from build123d import *

# Parameters (mm, degrees)
SKETCH1_W               = 800
SKETCH1_H               = 800
SKETCH1_W_2             = 700
SKETCH1_H_2             = 700
BOSS_EXTRUDE1_DEPTH     = 50
SKETCH2_W               = 50
SKETCH2_H               = 50
BOSS_EXTRUDE2_DEPTH     = 800
CUT_EXTRUDE1_DEPTH      = 980.795897113
CUT_EXTRUDE1_DEPTH_BACK = 980.795897113
SKETCH3_R               = 5


with BuildPart() as part:
    # Sketch1 → Boss-Extrude1 (new body)
    with BuildSketch(Plane(origin=(0, 0, 0), x_dir=(1, 0, 0), z_dir=(0, 1, 0))):
        Rectangle(SKETCH1_W, SKETCH1_H)
        Rectangle(SKETCH1_W_2, SKETCH1_H_2, mode=Mode.SUBTRACT)
    extrude(amount=BOSS_EXTRUDE1_DEPTH)

    # Sketch2 → Boss-Extrude2 (add)
    with BuildSketch(Plane.XZ.offset(-50)):
        with Locations((-375, 375)):
            Rectangle(SKETCH2_W, SKETCH2_H)
        with Locations((375, 375)):
            Rectangle(SKETCH2_W, SKETCH2_H)
        with Locations((375, -375)):
            Rectangle(SKETCH2_W, SKETCH2_H)
        with Locations((-375, -375)):
            Rectangle(SKETCH2_W, SKETCH2_H)
    extrude(amount=BOSS_EXTRUDE2_DEPTH)

    # Sketch3 → Cut-Extrude1 (cut, two sides: drawn at the far end of the back side and taken through both)
    with BuildSketch(Plane(origin=(0, 50, 0), x_dir=(1, 0, 0), z_dir=(0, 1, 0)).offset(-CUT_EXTRUDE1_DEPTH_BACK)):
        with Locations(Location((-200, 375, 0), (0, 0, 90))):
            Circle(SKETCH3_R)
        with Locations(Location((-375, 200, 0), (0, 0, 90))):
            Circle(SKETCH3_R)
        with Locations(Location((-375, -200, 0), (0, 0, 90))):
            Circle(SKETCH3_R)
        with Locations(Location((-200, -375, 0), (0, 0, 90))):
            Circle(SKETCH3_R)
        with Locations(Location((200, -375, 0), (0, 0, 90))):
            Circle(SKETCH3_R)
        with Locations(Location((375, -200, 0), (0, 0, 90))):
            Circle(SKETCH3_R)
        with Locations(Location((375, 200, 0), (0, 0, 90))):
            Circle(SKETCH3_R)
        with Locations(Location((200, 375, 0), (0, 0, 90))):
            Circle(SKETCH3_R)
    extrude(amount=CUT_EXTRUDE1_DEPTH + CUT_EXTRUDE1_DEPTH_BACK, mode=Mode.SUBTRACT)


solid = part.part
CAD build for the part. Positions are in the model's coordinates, mm. A direction names the side the tool comes from. Round coordinates to 2 decimals unless told otherwise and drop trailing zeros. Order: outer loops, then holes, each group sorted by start corner. A loop starts at its lowest first (then second) coordinate and runs counter-clockwise, first axis right, second up. Notation, with made-up numbers: (67, 68) - (102, 68) arc R8 cw to (102, 77) - close; hole circle Ø7 at (-32.75, 3.25). An arc over 180 degrees is marked (long way). Return JSON: item names as keys, results as strings.
(1) Cut at A-A (y = -82). Give the cut face in (x, z).
Answer key:
{"outline": "(-400, -400) - (-350, -400) - (-350, -350) - (-400, -350) - close; (-400, 350) - (-350, 350) - (-350, 400) - (-400, 400) - close; (350, -400) - (400, -400) - (400, -350) - (350, -350) - close; (350, 350) - (400, 350) - (400, 400) - (350, 400) - close"}
(2) Pull direction Z, two halves, no side cores. Call faces 5 (the face through (-2, 4, -400)), 6 (the face through (-357, 50, -2)), 7 (the face through (-375, 0, -5)), 8 (the face through (350, 25, 5)): +Z half, -Z half, draft (parallel to the pull), parting line (faces both ways), or undercut.
Answer key:
{"face 5": "-Z half", "face 6": "draft", "face 7": "undercut", "face 8": "undercut"}
(3) Pin check, flat tips, straight feed: pin 1 Ø15 at (x, z) = (-371.5, -52.5) entering from -Y; pin 2 Ø11.5 at (x, z) = (-375, -200) entering from +Y. Stop position of each tip, or through.
Answer key:
{"pin 1": "stops at y = 0", "pin 2": "stops at y = 50"}
(4) Cut at B-B (z = 55). Give the cut face in (x, y), then the cut area to 3 significant figures.
Answer key:
{"outline": "(-400, 0) - (-350, 0) - (-350, 50) - (-400, 50) - close; (350, 0) - (400, 0) - (400, 50) - (350, 50) - close", "area": "5,000 mm^2"}
(5) Wall check: probe 1 along Z at (x, y) = (-375, 24); probe 2 along X at (y, z) = (-564, -351). Give the ranges that are in metal, low to high. Write a range as from..to.
Answer key:
{"probe 1": "z = -400..-205, -195..195, 205..400", "probe 2": "x = -400..-350, 350..400"}
(6) Tool access for faces 1 (the face through (350, -370, 375)), 2 (the face through (-5, 25, -350)), 3 (the face through (-2, 4, 400)), 4 (the face through (-375, -370, -350)): list every direction of +Z, -Z, +X, -X, +Y, -Y with a clear straight run to the whole face (end or side of a thin tool).
Answer key:
{"face 1": "+Z, -Z, -Y", "face 2": "+Y, -Y", "face 3": "+Z, +X, -X, +Y, -Y", "face 4": "+X, -X, -Y"}
(7) Cut at C-C (x = -241.5). Give the cut face in (y, z).
Answer key:
{"outline": "(0, -400) - (50, -400) - (50, -350) - (0, -350) - close; (0, 350) - (50, 350) - (50, 400) - (0, 400) - close"}
